```python
from build123d import *

# Parameters (mm, degrees)
SKETCH_1_R       = 2.1
EXTRUDE_3_DEPTH  = 5
FILLET_1_R       = 5
CHAMFER_1_SIZE   = 2
CHAMFER_1_SIZE_2 = 2.97860662
CHAMFER_2_SIZE   = 4


with BuildPart() as part:
    # Эскиз1 → Бобышка-Вытянуть3 (new body)
    # profile 1 of 4: a face of its own
    with BuildSketch(Plane(origin=(0, 249.195974268, 0), x_dir=(1, 0, 0), z_dir=(0, 1, 0))):
        with BuildLine():
            ThreePointArc((100.251716198, -101.773129836), (97.92926953, -107.109956368), (94.808980694, -112.023129836))
            Line((94.808980694, -112.023129836), (88.058980694, -146.773129836))
            Line((88.058980694, -146.773129836), (100.251716198, -146.773129836))
            Line((100.251716198, -146.773129836), (100.251716198, -101.773129836))
        make_face()
    # profile 2 of 4: a face of its own
    with BuildSketch(Plane(origin=(0, 249.195974268, 0), x_dir=(1, 0, 0), z_dir=(0, 1, 0))):
        with BuildLine():
            Line((1.558980694, -138.773129836), (1.558980694, -146.773129836))
            Line((1.558980694, -146.773129836), (40.058980694, -146.773129836))
            Line((40.058980694, -146.773129836), (34.808980694, -112.023129836))
            ThreePointArc((34.808980694, -112.023129836), (28.511671278, -80.102125156), (49.53850264, -55.273129836))
            ThreePointArc((49.53850264, -55.273129836), (64.808980694, -52.023129836), (80.079458748, -55.273129836))
            ThreePointArc((80.079458748, -55.273129836), (92.976106795, -64.767059728), (100.735907579, -78.775761573))
            Line((100.735907579, -78.775761573), (100.735907579, -32.273129836))
            Line((100.735907579, -32.273129836), (1.558980694, -32.273129836))
            Line((1.558980694, -32.273129836), (1.558980694, -55.273129836))
            Line((1.558980694, -55.273129836), (17.308980694, -55.273129836))
            Line((17.308980694, -55.273129836), (17.308980694, -89.523129836))
            Line((17.308980694, -89.523129836), (17.308980694, -103.773129836))
            Line((17.308980694, -103.773129836), (28.308980694, -103.773129836))
            Line((28.308980694, -103.773129836), (28.308980694, -138.773129836))
            Line((28.308980694, -138.773129836), (1.558980694, -138.773129836))
        make_face()
        with Locations(Location((11.55898069, -40.273129836, 0), (0, 0, 180))):
            Circle(SKETCH_1_R, mode=Mode.SUBTRACT)
    # profile 3 of 4: a face of its own
    with BuildSketch(Plane(origin=(0, 249.195974268, 0), x_dir=(1, 0, 0), z_dir=(0, 1, 0))):
        Polygon((88.058980694, -160.773129836), (40.058980694, -160.773129836), (36.058980694, -160.773129836), (21.058980694, -152.773129836), (9.558980694, -152.773129836), (1.558980694, -146.773129836), (40.058980694, -146.773129836), (40.058980694, -152.773129836), (88.058980694, -152.773129836), align=None)
    # profile 4 of 4: a face of its own
    with BuildSketch(Plane(origin=(0, 249.195974268, 0), x_dir=(1, 0, 0), z_dir=(0, 1, 0))):
        with BuildLine():
            Line((88.058980694, -146.773129836), (88.058980694, -152.773129836))
            Line((88.058980694, -152.773129836), (88.058980694, -160.773129836))
            Line((88.058980694, -160.773129836), (92.058980694, -160.773129836))
            Line((92.058980694, -160.773129836), (107.058980694, -152.773129836))
            Line((107.058980694, -152.773129836), (120.058980694, -152.773129836))
            Line((120.058980694, -152.773129836), (128.058980694, -146.773129836))
            Line((128.058980694, -146.773129836), (128.058980694, -55.273129836))
            Line((128.058980694, -55.273129836), (128.058980694, -32.273129836))
            Line((128.058980694, -32.273129836), (107.058980694, -32.273129836))
            Line((107.058980694, -32.273129836), (100.735907579, -32.273129836))
            Line((100.735907579, -32.273129836), (100.735907579, -78.775761573))
            Line((100.735907579, -78.775761573), (107.058980694, -78.775761573))
            ThreePointArc((107.058980694, -78.775761573), (111.821891611, -90.274445705), (107.058980694, -101.773129836))
            Line((107.058980694, -101.773129836), (100.251716198, -101.773129836))
            Line((100.251716198, -101.773129836), (100.251716198, -146.773129836))
            Line((100.251716198, -146.773129836), (88.058980694, -146.773129836))
        make_face()
        with Locations(Location((118.058980694, -138.773129836, 0), (0, 0, 180))):
            Circle(SKETCH_1_R, mode=Mode.SUBTRACT)
        with Locations(Location((118.058980694, -40.273129836, 0), (0, 0, 180))):
            Circle(SKETCH_1_R, mode=Mode.SUBTRACT)
    extrude(amount=EXTRUDE_3_DEPTH)

    # Скругление1
    fillet_1_edges = [part.edges().sort_by_distance(p)[0] for p in [
        (28.308980694, 251.695974268, 103.773129836),
        (40.058980694, 251.695974268, 152.773129836),
        (88.058980694, 251.695974268, 152.773129836),
    ]]
    fillet(fillet_1_edges, radius=FILLET_1_R)

    # Фаска1
    # the kernel refuses this chamfer: 3.233771195, 2.97860662, 2 mm, written as the material it takes off along each edge
    with BuildSketch(Plane(origin=(100.251716198, 239.918924652, 101.773129836), x_dir=(-0.3715523502271027, -3.437549783964329e-15, 0.9284120050067838), z_dir=(0, 1, 0))) as chamfer_1_piece_1:
        with BuildLine():
            Line((3.591569227, 0), (-CHAMFER_1_SIZE * 0.371552350227, CHAMFER_1_SIZE * 0.928412005007))
            Line((-CHAMFER_1_SIZE * 0.371552350227, CHAMFER_1_SIZE * 0.928412005007), (0, 0))
            ThreePointArc((0, 0), (1.855343846, 0.04297528), (3.591569227, 0))
        make_face()
    extrude(amount=23.554099231, mode=Mode.SUBTRACT)
    with BuildSketch(Plane(origin=(100.735907579, 241.48601373, 78.775761573), x_dir=(-0.31276738664383585, -2.8936796166985435e-15, -0.9498297541412279), z_dir=(0, 1, 0))) as chamfer_1_piece_2:
        with BuildLine():
            Line((2.057201754, 0), (-CHAMFER_1_SIZE_2 * 0.312767386639, -CHAMFER_1_SIZE_2 * 0.949829754125))
            Line((-CHAMFER_1_SIZE_2 * 0.312767386639, -CHAMFER_1_SIZE_2 * 0.949829754125), (0, 0))
            ThreePointArc((0, 0), (1.071927906, -0.014084555), (2.057201754, 0))
        make_face()
    extrude(amount=20.419921076, mode=Mode.SUBTRACT)

    # Фаска2
    chamfer_2_edges = [part.edges().sort_by_distance(p)[0] for p in [
        (17.308980694, 251.695974268, 103.773129836),
    ]]
    chamfer(chamfer_2_edges, length=CHAMFER_2_SIZE)


solid = part.part
```
Input: part model. Units: mm. Frame: model coordinates. A direction names the side the tool comes from. Give positions to 0.01 mm unless a question says otherwise; leave off trailing zeros. Order: outer loops, then holes, each group sorted by start corner. A loop starts at its lowest first (then second) coordinate and runs counter-clockwise, first axis right, second up. Notation, with made-up numbers: (71, 8.25) -> (89, 8.25) arc R21 cw to (89, 32.25) -> close; hole circle Ø6 at (60.25, 31.25). An arc over 180 degrees is marked (long way). Write each question's results on one line, items separated by ' | '. Start each with the question number.
Item 1: Cut plane C-C on y = 252.3. Give the number of separate pieces and of enclosed holes in the cut face, then the cut area to 3 significant figures.
Item 2: Mould query, pull axis X, two halves, no side actions, for faces 5 (the flat face through (64, 252, 160.773)), 6 (the flat face through (19.281, 251.661, 101.745)), 7 (the cylindrical face through (97.078, 251.661, 108.627)). Classes: pulls with the +X half, pulls with the -X half, needs draft (parallel to the pull), parting line crosses it, or undercut.
Item 3: Line query: line 1 (Z direction, x = 10, y = 251.95); line 2 (Z direction, x = 11, y = 250.6); line 3 (Z direction, x = 26.5, y = 251.05) (3 decimals). Output: solid intervals per line, ascending.
Item 4: Set-up query: faces 1 (the flat face through (124.003, 251.661, 149.815)), 2 (the flat face through (15, 252, 152.773)), 3 (the flat face through (9, 252, 55.273)), 4 (the flat face through (37.47, 251.66, 129.64)). Return all of +Z, -Z, +X, -X, +Y, -Y with unobstructed straight access to the full face (end or side cutting, diameter ignored); none if empty.
Item 5: Contact query for flat-ended pins moving along their axis: P1, Ø1, axis at x = 22.5, y = 252.5, coming from the +Z side; P2, Ø2.5, axis at x = 118.06, z = 138.77, coming from the -Y side; P3, Ø0.8, axis at y = 250.5, z = 147.5, coming from the -X side; P4, Ø1.5, axis at y = 253, z = 118, coming from the -X side. Output: stop coordinate, or through.
Item 6: Cut plane A-A on z = 127.5. Return the cut outline in (x, y), then the cut area to 3 significant figures.
Item 7: Cut plane B-B on x = 96.5. Return the cut outline in (y, z).
Established:
1) separate pieces: 1 | enclosed holes: 4 | area: 7,870 mm^2
2) face 5: needs draft | face 6: pulls with the -X half | face 7: undercut
3) line 1: 32.27 to 38.87, 41.68 to 55.27, 138.77 to 152.77 | line 2: 32.27 to 38.25, 42.3 to 55.27, 138.77 to 152.77 | line 3: 32.273 to 104.924, 138.773 to 155.675
4) face 1: +Z, +X, +Y, -Y | face 2: +Z, -X, +Y, -Y | face 3: -X, +Y, -Y | face 4: +Y, -Y
5) P1: z = 153.81 | P2: through | P3: x = 1.99 | P4: x = 28.31
6) outline: (28.31, 249.2) -> (37.15, 249.2) -> (37.15, 254.2) -> (28.31, 254.2) -> close; (91.8, 249.2) -> (128.06, 249.2) -> (128.06, 254.2) -> (91.8, 254.2) -> close | area: 225 mm^2
7) outline: (249.2, 32.27) -> (254.2, 32.27) -> (254.2, 69.47) -> (249.2, 69.47) -> close; (249.2, 109.57) -> (254.2, 109.57) -> (254.2, 158.4) -> (249.2, 158.4) -> close
